Input: part model. Units: mm. Frame: model coordinates. Face numbers are marked on the shaded views. A direction names the side the tool comes from. Coordinates: 2 decimals unless noted, no trailing zeros. Loops run counter-clockwise (first coordinate to the right, second up) from the corner with the lowest first, then second, coordinate; pieces in that order, holes last.
Item 1: Reachability of the marked faces 1 and 2 from +Z, -Z, +X, -X, +Y, -Y: full face, straight path, thin tool, end or side. Return the list, or none.
Item 2: Pull-direction query (X, two-part tool) for the marked faces 3, 4 and 5; classes: released by +X, released by -X, zero draft, split by the parting line, or undercut.
Item 3: Contact query for flat-ended pins moving along their axis: P1, Ø14.5, axis at x = -26.5, y = -41, coming from the +Z side; P2, Ø2, axis at y = -30.5, z = 1, coming from the +X side; P3, Ø4, axis at y = -30.5, z = 1, coming from the +X side; P4, Ø4, axis at x = 9.5, z = 5.5, coming from the -Y side. Output: stop coordinate, or through.
Item 4: Section B-B on y = -28.5. Return loops of the section in (x, z).
Item 5: Ray query, line 1 along Y through (x, z) = (-3, 0.75); line 2 along X through (y, z) = (-10, 0.5); line 3 along X through (y, z) = (-21, 1). Return the intervals inside material, ascending.
Item 6: Section C-C on x = -25.5. Return loops of the section in (y, z).
Item 7: Section A-A on x = 0. Return loops of the section in (y, z), and give its area (3 significant figures).
Item 8: Section D-D on y = -36. Give the number of separate pieces and of enclosed holes in the cut face, and give its area (3 significant figures).
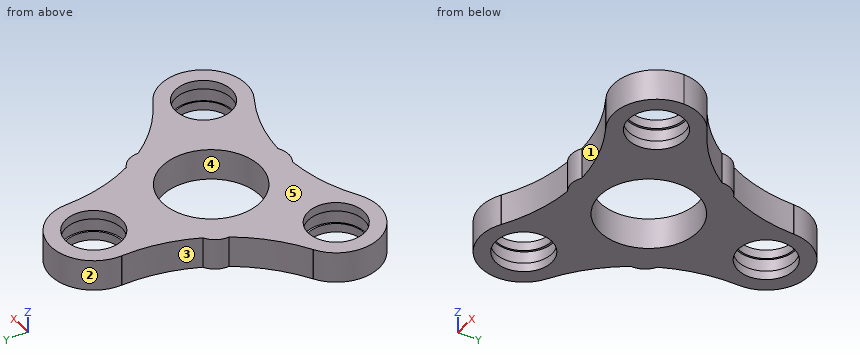
```python
from build123d import *

# Parameters (mm, degrees)
F0_R     = 6.2993
F0_R_2   = 11
F1_DEPTH = 7
F4_R     = 6.6710532067
F5_DEPTH = 3


# Not quite as in the source:
# - ends of sketch curves that miss each other by under 0.0002 mm in the source are joined
# - a feature names something its author has since deleted; it is built from what else it names


with BuildPart() as f1:
    # F0 (on Top) → F1 (new body)
    with BuildSketch(Plane.XY):
        with BuildLine():
            ThreePointArc((9.6625090534, -0.0929069647), (9.6627025372, -0.0464533389), (9.6629557026, 0))
            ThreePointArc((9.6629557026, 0), (0, 9.6629557026), (-9.6629557026, 0))
            ThreePointArc((-9.6629557026, 0), (-9.662702535, -0.0464535369), (-9.6625090496, -0.0929073607))
            ThreePointArc((-9.6625090496, -0.0929073607), (1.98e-07, -9.6629557026), (9.6625090534, -0.0929069647))
        make_face()
        Circle(F0_R, mode=Mode.SUBTRACT)
        with BuildLine():
            ThreePointArc((-13.4378241011, -40.0117243144), (-18.2291272521, -31.6666830127), (-27.8515741938, -31.5972923328))
            ThreePointArc((-27.8515741938, -31.5972923328), (-27.8919011281, -31.6203516814), (-27.9322576549, -31.6433592003))
            ThreePointArc((-27.9322576549, -31.6433592003), (-31.4691449177, -44.8432021657), (-18.2693019524, -48.3800894285))
            ThreePointArc((-18.2693019524, -48.3800894285), (-18.2291987635, -48.3566435113), (-18.1890654853, -48.3332491365))
            ThreePointArc((-18.1890654853, -48.3332491365), (-14.7092843829, -44.8029159735), (-13.4378241011, -40.0117243144))
        make_face()
        with Locations((-23.1007798037, -40.0117243144)):
            Circle(F0_R, mode=Mode.SUBTRACT)
        with BuildLine():
            ThreePointArc((27.9322576549, -31.6433592003), (27.8919013007, -31.6203517785), (27.8515745387, -31.5972925275))
            ThreePointArc((27.8515745387, -31.5972925275), (14.7324146896, -35.1802464631), (18.1890654853, -48.3332491365))
            ThreePointArc((18.1890654853, -48.3332491365), (18.2291987635, -48.3566435113), (18.2693019524, -48.3800894285))
            ThreePointArc((18.2693019524, -48.3800894285), (27.9322576549, -48.3800894285), (32.7637355062, -40.0117243144))
            ThreePointArc((32.7637355062, -40.0117243144), (31.4691449177, -35.1802464631), (27.9322576549, -31.6433592003))
        make_face()
        with Locations((23.1007798037, -40.0117243144)):
            Circle(F0_R, mode=Mode.SUBTRACT)
        with BuildLine():
            ThreePointArc((13.3320983645, -16.0921664972), (10.5773906807, -8.3035279339), (9.6625090534, -0.0929069647))
            ThreePointArc((9.6625090534, -0.0929069647), (1.98e-07, -9.6629557026), (-9.6625090496, -0.0929073607))
            ThreePointArc((-9.6625090496, -0.0929073607), (-10.5773905595, -8.3035281796), (-13.3320981392, -16.0921666073))
            ThreePointArc((-13.3320981392, -16.0921666073), (-14.506503102, -18.2991494053), (-15.8306037894, -20.4197053365))
            ThreePointArc((-15.8306037894, -20.4197053365), (-21.1984087389, -26.6996712943), (-27.8515741938, -31.5972923328))
            ThreePointArc((-27.8515741938, -31.5972923328), (-18.2291272521, -31.6666830127), (-13.4378241011, -40.0117243144))
            ThreePointArc((-13.4378241011, -40.0117243144), (-14.7092843829, -44.8029159735), (-18.1890654853, -48.3332491365))
            ThreePointArc((-18.1890654853, -48.3332491365), (-10.6210183315, -45.0202493827), (-2.4985056329, -43.5115769352))
            ThreePointArc((-2.4985056329, -43.5115769352), (0, -43.4251500733), (2.4985056329, -43.5115769352))
            ThreePointArc((2.4985056329, -43.5115769352), (10.6210183315, -45.0202493827), (18.1890654853, -48.3332491365))
            ThreePointArc((18.1890654853, -48.3332491365), (14.7324146896, -35.1802464631), (27.8515745387, -31.5972925275))
            ThreePointArc((27.8515745387, -31.5972925275), (21.1984090122, -26.6996713122), (15.8306039974, -20.4197051964))
            ThreePointArc((15.8306039974, -20.4197051964), (14.506503323, -18.2991492777), (13.3320983645, -16.0921664972))
        make_face()
        with Locations((0, -26.6744828763)):
            Circle(F0_R_2, mode=Mode.SUBTRACT)
        with BuildLine():
            ThreePointArc((15.8306039974, -20.4197051964), (15.223256939, -17.8853313846), (13.3320983645, -16.0921664972))
            ThreePointArc((13.3320983645, -16.0921664972), (14.506503323, -18.2991492777), (15.8306039974, -20.4197051964))
        make_face()
        with BuildLine():
            ThreePointArc((-15.8306037894, -20.4197053365), (-14.506503102, -18.2991494053), (-13.3320981392, -16.0921666073))
            ThreePointArc((-13.3320981392, -16.0921666073), (-15.223256939, -17.8853313846), (-15.8306037894, -20.4197053365))
        make_face()
        with BuildLine():
            ThreePointArc((-2.4985056329, -43.5115769352), (0, -44.2527858596), (2.4985056329, -43.5115769352))
            ThreePointArc((2.4985056329, -43.5115769352), (0, -43.4251500733), (-2.4985056329, -43.5115769352))
        make_face()
    extrude(amount=F1_DEPTH)

    # F4 (on line) → F5 (cut)
    with BuildSketch(Plane.XY.offset(2)):
        Circle(F4_R)
        with Locations((-23.0745827089, -39.8926408961)):
            Circle(F4_R)
        with Locations((23.0107490857, -39.9294952557)):
            Circle(F4_R)
    extrude(amount=F5_DEPTH, mode=Mode.SUBTRACT)


solid = f1.part
```
Results found:
1. face 1: +Z, -Z, -Y
1. face 2: +Z, -Z, +Y
2. face 3: released by -X
2. face 4: undercut
2. face 5: zero draft
3. P1: stops at z = 7
3. P2: stops at x = 27.68
3. P3: stops at x = 29.18
3. P4: stops at y = -45.3
4. outline: (-23.29, 0) - (-10.85, 0) - (-10.85, 7) - (-23.29, 7) - close; (10.85, 0) - (23.29, 0) - (23.29, 7) - (10.85, 7) - close
5. line 1: y = -43.55 to -37.26, -16.09 to -5.54, 5.54 to 9.19
5. line 2: x = -11.01 to 11.01
5. line 3: x = -16.23 to -9.42, 9.42 to 16.23
6. outline: (-49.37, 0) - (-45.84, 0) - (-45.84, 2) - (-46.11, 2) - (-46.11, 5) - (-45.84, 5) - (-45.84, 7) - (-49.37, 7) - close; (-34.19, 0) - (-30.13, 0) - (-30.13, 7) - (-34.19, 7) - (-34.19, 5) - (-33.68, 5) - (-33.68, 2) - (-34.19, 2) - close
7. outline: (-44.25, 0) - (-37.67, 0) - (-37.67, 7) - (-44.25, 7) - close; (-15.67, 0) - (-6.3, 0) - (-6.3, 2) - (-6.67, 2) - (-6.67, 5) - (-6.3, 5) - (-6.3, 7) - (-15.67, 7) - close; (6.3, 0) - (9.66, 0) - (9.66, 7) - (6.3, 7) - (6.3, 5) - (6.67, 5) - (6.67, 2) - (6.3, 2) - close
7. area: 133 mm2
8. separate pieces: 4
8. enclosed holes: 0
8. area: 222 mm2
